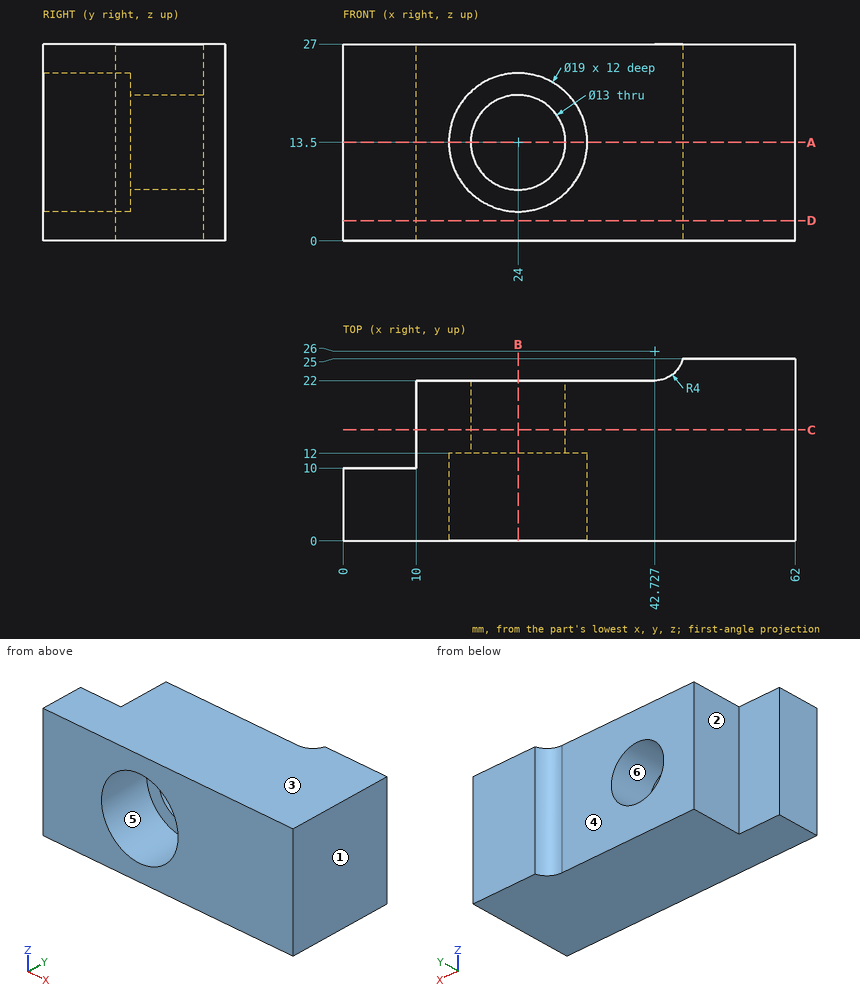
Print and shaded views of the part. All mm, measured from the part's lowest x, y and z. A direction names the side the tool comes from. Coordinates: 2 decimals unless noted, no trailing zeros. Loops run counter-clockwise (first coordinate to the right, second up) from the corner with the lowest first, then second, coordinate; pieces in that order, holes last. Notation, with made-up numbers: (82, 33.25) -> (96, 33.25) arc R11 cw to (96, 49.25) -> close; hole circle Ø11 at (83.25, 48.25). An arc over 180 degrees is marked (long way). Use a Markdown table: item, result. Add a question column.
Item 1: Pull direction Z, two halves, no side cores. Call the marked faces 3, 4, 5 and 6: +Z half, -Z half, draft (parallel to the pull), parting line (faces both ways), or undercut.
Item 2: Probe probe 1 along Z at (x, y) = (24, 3); probe 2 along Y at (x, z) = (5.5, 25); probe 3 along Y at (x, z) = (31.5, 8.5). List the from-to ranges inside material, lowest first.
Item 3: Band-saw the part on B-B on x = 24. Write the cut outline in (y, z), plus the area to 3 significant figures.
Item 4: Flat gauge pins, fed straight in: P1, Ø6, axis at x = 8, z = 21.5, coming from the +Y side; P2, Ø3.5, axis at y = 17, z = 19, coming from the -X side; P3, Ø2, axis at x = 22, z = 22.5, coming from the -Y side. Where does each tip first touch, or does it go through?
Item 5: Which spindle directions (+Z, -Z, +X, -X, +Y, -Y) get a long thin tool onto all of the face, cutting with end or side? Do the marked faces 1 and 2. Say none if no direction does.
Item 6: Band-saw the part on C-C on y = 15.25. Write the cut outline in (x, z), plus the area to 3 significant figures.
Item 7: Band-saw the part on D-D on z = 2.75. Write the cut outline in (x, y).
Item 8: Band-saw the part on A-A on z = 13.5. Write the cut outline in (x, y).
Geometry says:
| question | item | result |
|---|---|---|
| 1 | face 3 | +Z half |
| 1 | face 4 | draft |
| 1 | face 5 | undercut |
| 1 | face 6 | undercut |
| 2 | probe 1 | 0 to 4, 23 to 27 |
| 2 | probe 2 | 0 to 10 |
| 2 | probe 3 | 12 to 22 |
| 3 | outline | (0, 0) -> (22, 0) -> (22, 7) -> (12, 7) -> (12, 4) -> (0, 4) -> close; (0, 23) -> (12, 23) -> (12, 20) -> (22, 20) -> (22, 27) -> (0, 27) -> close |
| 3 | area | 236 mm² |
| 4 | P1 | y = 22 |
| 4 | P2 | x = 10 |
| 4 | P3 | y = 0 |
| 5 | face 1 | +Z, -Z, +X, +Y, -Y |
| 5 | face 2 | +Z, -Z, -X, +Y |
| 6 | outline | (10, 0) -> (62, 0) -> (62, 27) -> (10, 27) -> close; hole circle Ø13 at (24, 13.5) |
| 6 | area | 1,270 mm² |
| 7 | outline | (0, 0) -> (62, 0) -> (62, 25) -> (46.6, 25) arc R4 cw to (42.73, 22) -> (10, 22) -> (10, 10) -> (0, 10) -> close |
| 8 | outline | (0, 0) -> (14.5, 0) -> (14.5, 12) -> (17.5, 12) -> (17.5, 22) -> (10, 22) -> (10, 10) -> (0, 10) -> close; (30.5, 12) -> (33.5, 12) -> (33.5, 0) -> (62, 0) -> (62, 25) -> (46.6, 25) arc R4 cw to (42.73, 22) -> (30.5, 22) -> close |
